```python
from build123d import *

# Parameters (mm, degrees)
BOSS_EXTRUDE1_DEPTH      = 10
BOSS_EXTRUDE1_DEPTH_BACK = 10
SKETCH1_R                = 9
BOSS_EXTRUDE2_DEPTH      = 9
BOSS_EXTRUDE2_DEPTH_BACK = 9
BOSS_EXTRUDE4_DEPTH      = 5
BOSS_EXTRUDE4_DEPTH_BACK = 5
BOSS_EXTRUDE3_DEPTH      = 10
BOSS_EXTRUDE3_DEPTH_BACK = 30
SKETCH2_W                = 5
SKETCH2_H                = 20
SKETCH6_W                = 30
SKETCH6_H                = 5
BOSS_EXTRUDE6_DEPTH      = 10
FILLET1_R                = 10
M5_CLEARANCE_HOLE1_D     = 5.5


with BuildPart() as part:
    # Sketch1 → Boss-Extrude1 (new, two sides: drawn at the far end of the back side and taken through both)
    with BuildSketch(Plane(origin=(0, 0, 0), x_dir=(1, 0, 0), z_dir=(0, 1, 0)).offset(-BOSS_EXTRUDE1_DEPTH_BACK)):
        with BuildLine():
            Line((-9.406779661, -11.355932203), (-9.406779661, 8.644067797))
            Line((-9.406779661, 8.644067797), (-14.406779661, 8.644067797))
            Line((-14.406779661, 8.644067797), (-14.406779661, -56.355932203))
            ThreePointArc((-14.406779661, -56.355932203), (0.593220339, -71.355932203), (15.593220339, -56.355932203))
            Line((15.593220339, -56.355932203), (15.593220339, 8.644067797))
            Line((15.593220339, 8.644067797), (10.593220339, 8.644067797))
            Line((10.593220339, 8.644067797), (10.593220339, -11.355932203))
            Line((10.593220339, -11.355932203), (-9.406779661, -11.355932203))
        make_face()
        with Locations(Location((0.593220339, -56.355932203, 0), (0, 0, 270))):
            Circle(SKETCH1_R, mode=Mode.SUBTRACT)
    extrude(amount=BOSS_EXTRUDE1_DEPTH + BOSS_EXTRUDE1_DEPTH_BACK)

    # Sketch1<3> → Boss-Extrude2 (add, two sides: drawn at the far end of the back side and taken through both)
    # profile 1 of 2: a face of its own
    with BuildSketch(Plane(origin=(0, 0, 0), x_dir=(1, 0, 0), z_dir=(0, 1, 0)).offset(-BOSS_EXTRUDE2_DEPTH_BACK)):
        with BuildLine():
            ThreePointArc((9.593220339, -56.355932203), (6.95718137, -49.991971173), (0.593220339, -47.355932203))
            ThreePointArc((0.593220339, -47.355932203), (-5.770740692, -62.719893234), (9.593220339, -56.355932203))
        make_face()
        with BuildLine():
            ThreePointArc((8.593220339, -56.355932203), (-5.063633911, -62.012786453), (0.593220339, -48.355932203))
            ThreePointArc((0.593220339, -48.355932203), (6.250074588, -50.699077954), (8.593220339, -56.355932203))
        make_face(mode=Mode.SUBTRACT)
    # profile 2 of 2: a face of its own
    with BuildSketch(Plane(origin=(0, 0, 0), x_dir=(1, 0, 0), z_dir=(0, 1, 0)).offset(-BOSS_EXTRUDE2_DEPTH_BACK)):
        with BuildLine():
            ThreePointArc((9.593220339, -56.355932203), (6.95718137, -49.991971173), (0.593220339, -47.355932203))
            ThreePointArc((0.593220339, -47.355932203), (-5.770740692, -62.719893234), (9.593220339, -56.355932203))
        make_face()
        with BuildLine():
            ThreePointArc((8.593220339, -56.355932203), (-5.063633911, -62.012786453), (0.593220339, -48.355932203))
            ThreePointArc((0.593220339, -48.355932203), (6.250074588, -50.699077954), (8.593220339, -56.355932203))
        make_face(mode=Mode.SUBTRACT)
    extrude(amount=BOSS_EXTRUDE2_DEPTH + BOSS_EXTRUDE2_DEPTH_BACK)

    # Sketch1<4> → Boss-Extrude4 (add, two sides: drawn at the far end of the back side and taken through both)
    # profile 1 of 2: a face of its own
    with BuildSketch(Plane(origin=(0, 0, 0), x_dir=(1, 0, 0), z_dir=(0, 1, 0)).offset(-BOSS_EXTRUDE4_DEPTH_BACK)):
        with BuildLine():
            ThreePointArc((8.593220339, -56.355932203), (6.250074588, -50.699077954), (0.593220339, -48.355932203))
            ThreePointArc((0.593220339, -48.355932203), (-5.063633911, -62.012786453), (8.593220339, -56.355932203))
        make_face()
        with BuildLine():
            ThreePointArc((5.093220339, -56.355932203), (-2.588760176, -59.537912719), (0.593220339, -51.855932203))
            ThreePointArc((0.593220339, -51.855932203), (3.775200854, -53.173951688), (5.093220339, -56.355932203))
        make_face(mode=Mode.SUBTRACT)
    # profile 2 of 2: a face of its own
    with BuildSketch(Plane(origin=(0, 0, 0), x_dir=(1, 0, 0), z_dir=(0, 1, 0)).offset(-BOSS_EXTRUDE4_DEPTH_BACK)):
        with BuildLine():
            ThreePointArc((8.593220339, -56.355932203), (6.250074588, -50.699077954), (0.593220339, -48.355932203))
            ThreePointArc((0.593220339, -48.355932203), (-5.063633911, -62.012786453), (8.593220339, -56.355932203))
        make_face()
        with BuildLine():
            ThreePointArc((5.093220339, -56.355932203), (-2.588760176, -59.537912719), (0.593220339, -51.855932203))
            ThreePointArc((0.593220339, -51.855932203), (3.775200854, -53.173951688), (5.093220339, -56.355932203))
        make_face(mode=Mode.SUBTRACT)
    extrude(amount=BOSS_EXTRUDE4_DEPTH + BOSS_EXTRUDE4_DEPTH_BACK)

    # Sketch2 → Boss-Extrude3 (add, two sides: drawn at the far end of the back side and taken through both)
    with BuildSketch(Plane(origin=(0, 10, 0), x_dir=(1, 0, 0), z_dir=(0, 1, 0)).offset(-BOSS_EXTRUDE3_DEPTH_BACK)):
        with Locations((13.093220339, -1.355932203)):
            Rectangle(SKETCH2_W, SKETCH2_H)
        with Locations((-11.906779661, -1.355932203)):
            Rectangle(SKETCH2_W, SKETCH2_H)
    extrude(amount=BOSS_EXTRUDE3_DEPTH + BOSS_EXTRUDE3_DEPTH_BACK)

    # Sketch6 → Boss-Extrude6 (add)
    with BuildSketch(Plane(origin=(0, 10, 0), x_dir=(1, 0, 0), z_dir=(0, 1, 0))):
        with Locations((0.593220339, -13.855932203)):
            Rectangle(SKETCH6_W, SKETCH6_H)
    extrude(amount=BOSS_EXTRUDE6_DEPTH)

    # Fillet1
    fillet1_edges = [part.edges().sort_by_distance(p)[0] for p in [
        (-11.906779661, -10, 11.355932203),
        (13.093220339, -10, 11.355932203),
    ]]
    fillet(fillet1_edges, radius=FILLET1_R - 0.0001)  # a hair under: the kernel refuses the full size

    # M5 Clearance Hole1 (through all)
    with Locations(Plane.XY.offset(16.355932203)):
        with Locations((0.593220339, 15)):
            Hole(M5_CLEARANCE_HOLE1_D / 2)


solid = part.part
```
The listing builds one solid part. Answer for the finished solid, in the listing's coordinates (mm). A direction names the side the tool comes from. Round coordinates to 2 decimals unless told otherwise and drop trailing zeros. Write each loop counter-clockwise with the first axis right and the second up, starting at its lowest first coordinate (ties: lowest second). Pieces come first, ordered by that corner, then holes. Notation, with made-up numbers: (73.25, 6) -> (115.25, 6) arc R19 cw to (115.25, 42) -> close; hole circle Ø6 at (56, -18). An arc over 180 degrees is marked (long way). Write item = value, one per line.
1) Section B-B on y = 0.5 is taken. Write down the section's boundary in (x, z).
Check values:
outline = (-14.41, -8.64) -> (-9.41, -8.64) -> (-9.41, 11.36) -> (10.59, 11.36) -> (10.59, -8.64) -> (15.59, -8.64) -> (15.59, 56.36) arc R15 ccw to (-14.41, 56.36) -> close; hole circle Ø9 at (0.59, 56.36)
2) Section D-D on z = 23.5 is taken. Write down the section's boundary in (x, y).
Check values:
outline = (-14.41, -10) -> (15.59, -10) -> (15.59, 10) -> (-14.41, 10) -> close
3) Given pin 1 (12 mm diameter, centred on x = -6, y = 11, fed in from +Z); pin 2 (12 mm diameter, centred on x = -6, z = 61, fed in from -Y); pin 3 (8 mm diameter, centred on x = 0.59, z = 56.36, fed in from +Y); pin 4 (9 mm diameter, centred on x = -1.5, z = 53, fed in from +Y), each flat-ended and moving along its own axis, determine where each tip first touches the part or whether it passes through.
Check values:
pin_1 = 71.34
pin_2 = -10
pin_3 = through
pin_4 = 9
4) For a pull along Z with two mould halves and no side action, classify faces 4 (the flat face through (4, 15, 16.356)), 5 (the flat face through (13, 0, -8.644)), 6 (the cylindrical face through (0.951, 17.727, 13.821)), 7 (the cylindrical face through (3.3, 9.49, 64.94)) as released by +Z, released by -Z, zero draft, split by the parting line, or undercut.
Check values:
face_4 = released by +Z
face_5 = released by -Z
face_6 = zero draft
face_7 = undercut
5) Straight lines are drawn through the part: line 1 along X through (y, z) = (10.5, 6.5); line 2 along Y through (x, z) = (4, 20); line 3 along Z through (x, y) = (-6.5, 18). For each, find the intervals that lie inside material, in ascending order. Write a range as [from, to].
Check values:
line_1 = [-14.41, -9.41], [10.59, 15.59]
line_2 = [-10, 10]
line_3 = [11.36, 16.36]
6) Which of the six approach directions +Z, -Z, +X, -X, +Y, -Y give full straight-line access (tool end or side, diameter ignored) to faces 1 (the flat face through (4, -5, 60)), 2 (the flat face through (4, 5, 60)), 3 (the flat face through (-12, -20, 1))?
Check values:
face_1 = -Y
face_2 = +Y
face_3 = +Z, -Z, +X, -X, -Y
7) Section A-A on y = 15 is taken. Write down the section's boundary in (x, z).
Check values:
outline = (-14.41, -8.64) -> (-9.41, -8.64) -> (-9.41, 11.36) -> (-2.16, 11.36) -> (-2.16, 16.36) -> (-14.41, 16.36) -> close; (3.34, 11.36) -> (10.59, 11.36) -> (10.59, -8.64) -> (15.59, -8.64) -> (15.59, 16.36) -> (3.34, 16.36) -> close
8) Section C-C on z = 58.5 is taken. Write down the section's boundary in (x, y), plus the area to 3 significant figures.
Check values:
outline = (-14.25, -10) -> (-8.15, -10) -> (-8.15, -9) -> (-7.11, -9) -> (-7.11, -5) -> (-3.36, -5) -> (-3.36, 5) -> (-7.11, 5) -> (-7.11, 9) -> (-8.15, 9) -> (-8.15, 10) -> (-14.25, 10) -> close; (4.55, -5) -> (8.3, -5) -> (8.3, -9) -> (9.33, -9) -> (9.33, -10) -> (15.44, -10) -> (15.44, 10) -> (9.33, 10) -> (9.33, 9) -> (8.3, 9) -> (8.3, 5) -> (4.55, 5) -> close
area = 356 mm²
